The drawing under review shows one solid part. Ordinate dimensions are in mm from its lowest x, y, z. A direction names the side the tool comes from. Give positions to 0.01 mm unless a question says otherwise; leave off trailing zeros. Write each loop counter-clockwise with the first axis right and the second up, starting at its lowest first coordinate (ties: lowest second). Pieces come first, ordered by that corner, then holes. Notation, with made-up numbers: M 87,-9.5 L 121,-9.5 A29 cw 121,10.5 Z; hole C 54.5,30 d1. An arc over 180 degrees is marked long. Write item = value, one per line. Start each with the question number.
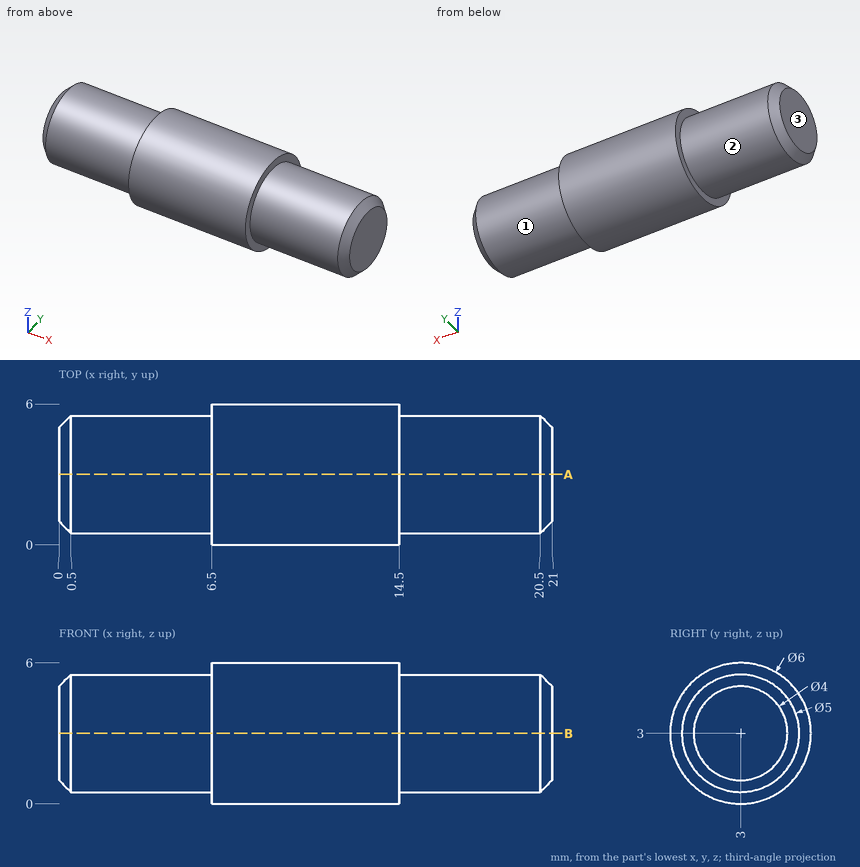
Item 1: To check wall thickness, follow probe 1 along Z at (x, y) = (17.5, 3); probe 2 along X at (y, z) = (5.1, 1.35); probe 3 along X at (y, z) = (1.3, 4.7). State the ranges of each line that lie inside material, in increasing order. Write a range as [from, to].
Item 2: Clearance check with flat-ended pins moving along their axes: P1, Ø1.5, axis at x = 4.5, y = 2, coming from the -Z side; P2, Ø2, axis at x = 14.5, z = 4.5, coming from the -Y side. State where each tip first meets the part, or that it passes through.
Item 3: For the marked faces 1, 2 and 3, list the 3-axis set-ups (+Z, -Z, +X, -X, +Y, -Y) from which the entire face can be reached by the end or side of a thin tool; tool diameter is ignored.
Item 4: We need section A-A, the plane y = 3. Write out the cut boundary in (x, z).
Worked out:
q1.probe_1 = [0.5, 5.5]
q1.probe_2 = [6.5, 14.5]
q1.probe_3 = [0.4, 20.6]
q2.P1 = 0.51
q2.P2 = 0.04
q3.face_1 = +X
q3.face_2 = -X
q3.face_3 = +Z, -Z, -X, +Y, -Y
q4.outline = M 0,1 L 0.5,0.5 L 6.5,0.5 L 6.5,0 L 14.5,0 L 14.5,0.5 L 20.5,0.5 L 21,1 L 21,5 L 20.5,5.5 L 14.5,5.5 L 14.5,6 L 6.5,6 L 6.5,5.5 L 0.5,5.5 L 0,5 Z
